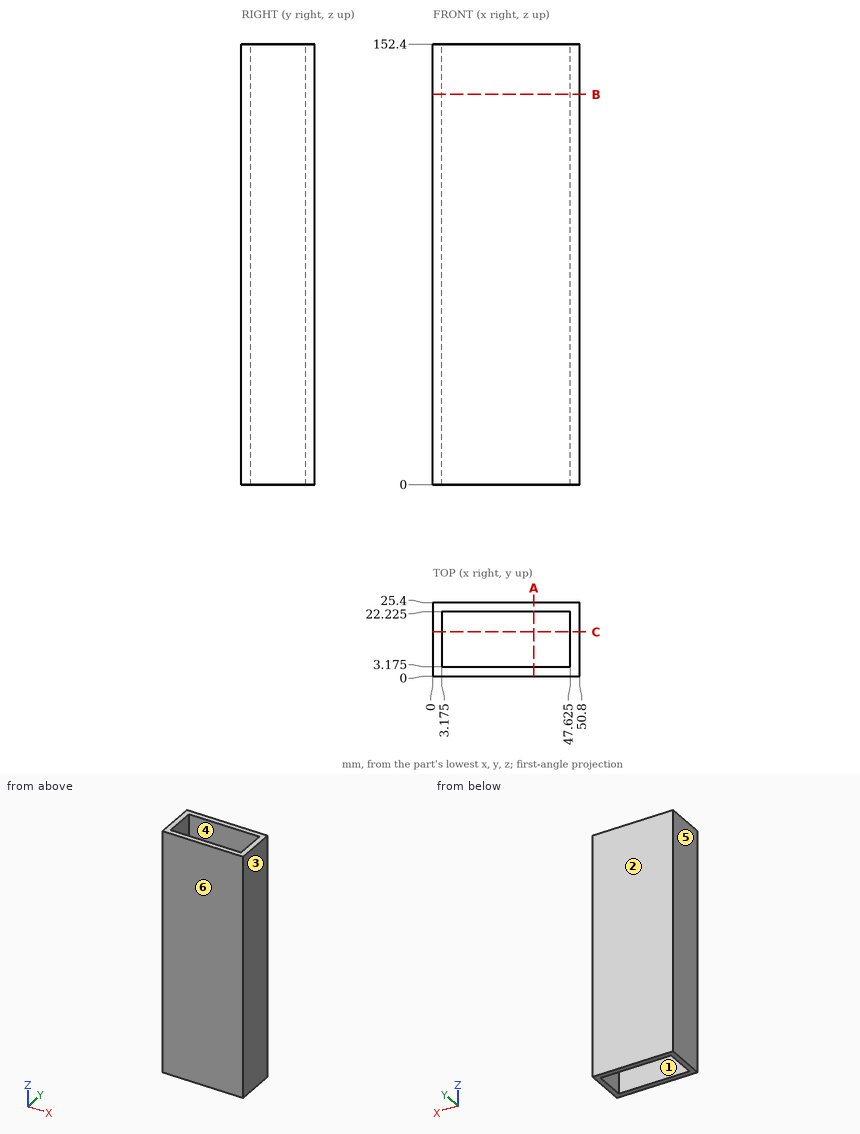
Study the drawing (mm; zero at the part's minimum x, y, z) and answer. A direction names the side the tool comes from. Coordinates: 2 decimals unless noted, no trailing zeros. Loops run counter-clockwise (first coordinate to the right, second up) from the corner with the lowest first, then second, coordinate; pieces in that order, holes last. Notation, with made-up numbers: (43, 30) -> (102, 30) arc R14 cw to (102, 45) -> close; hole circle Ø6 at (39, 42). An arc over 180 degrees is marked (long way). Write each question's results on one line, items separated by ' | '. Start each with the question number.
1) For the marked faces 1 and 2, determine the directions among +Z, -Z, +X, -X, +Y, -Y from which every point of the face is accessible in a straight line to the end or side of a thin tool.
2) The mould has two halves that part along X. Classify the marked faces 3, 4, 5 and 6: pulls with the +X half, pulls with the -X half, needs draft (parallel to the pull), parting line crosses it, or undercut.
3) Find section B-B on z = 135. Determine the outline of the cut face in (x, y) (3 decimals), then the cut area to 3 significant figures.
4) Find section A-A on x = 35. Determine the outline of the cut face in (y, z) (3 decimals).
5) A flat-ended cylindrical pin translates along its axis: P1, Ø22, axis at x = 21.5, z = 62.5, coming from the -Y side. Find the tip coordinate at first contact, or state that the pin passes through.
6) Find section C-C on y = 15.25. Determine the outline of the cut face in (x, z) (3 decimals).
7) Consider line 1 along X through (y, z) = (15.5, 90) (3 decimals); line 2 along Y through (x, z) = (35, 116.5) (3 decimals). Determine where each line is inside the solid, lowest interval first.
Response values:
1) face 1: +Z, -Z | face 2: +Z, -Z, +X, -X, +Y
2) face 3: pulls with the +X half | face 4: undercut | face 5: pulls with the -X half | face 6: needs draft
3) outline: (0, 0) -> (50.8, 0) -> (50.8, 25.4) -> (0, 25.4) -> close; hole (3.175, 3.175) -> (47.625, 3.175) -> (47.625, 22.225) -> (3.175, 22.225) -> close | area: 444 mm^2
4) outline: (0, 0) -> (3.175, 0) -> (3.175, 152.4) -> (0, 152.4) -> close; (22.225, 0) -> (25.4, 0) -> (25.4, 152.4) -> (22.225, 152.4) -> close
5) P1: stops at y = 0
6) outline: (0, 0) -> (3.175, 0) -> (3.175, 152.4) -> (0, 152.4) -> close; (47.625, 0) -> (50.8, 0) -> (50.8, 152.4) -> (47.625, 152.4) -> close
7) line 1: x = 0 to 3.175, 47.625 to 50.8 | line 2: y = 0 to 3.175, 22.225 to 25.4
